The model under review builds one solid part; all positions refer to its coordinate system, in mm. Coordinates: 2 decimals unless noted, no trailing zeros. Loops run counter-clockwise (first coordinate to the right, second up) from the corner with the lowest first, then second, coordinate; pieces in that order, holes last. Notation, with made-up numbers: M -5,41 L 49,41 A31 cw 49,77 Z; hole C 21,20 d7. An arc over 180 degrees is marked long. Return JSON: item names as keys, results as strings.
```python
from build123d import *

# Parameters (mm, degrees)
SKETCH1_W           = 50
SKETCH1_H           = 23.75
BOSS_EXTRUDE1_DEPTH = 4
FILLET1_R           = 1.5
SKETCH2_R           = 1.8
CUT_EXTRUDE1_DEPTH  = 28.964542281


with BuildPart() as part:
    # Sketch1 → Boss-Extrude1 (new body)
    with BuildSketch(Plane.XY):
        Rectangle(SKETCH1_W, SKETCH1_H)
    extrude(amount=BOSS_EXTRUDE1_DEPTH)

    # Fillet1
    fillet1_edges = [part.edges().sort_by_distance(p)[0] for p in [
        (-25, 11.875, 2),
        (25, 11.875, 2),
    ]]
    fillet(fillet1_edges, radius=FILLET1_R)

    # Sketch2 → Cut-Extrude1 (cut, through all)
    with BuildSketch(Plane.XY.offset(4)):
        with Locations((-12.75, -1.625)):
            Circle(SKETCH2_R)
        with Locations((-20, 8.375)):
            Circle(SKETCH2_R)
        with Locations((12.75, -1.625)):
            Circle(SKETCH2_R)
        with Locations((20, 8.375)):
            Circle(SKETCH2_R)
    extrude(amount=-CUT_EXTRUDE1_DEPTH, mode=Mode.SUBTRACT)


solid = part.part
```
1. Add section B-B on z = 3.35. Give the boundary of the cut face in (x, y) (3 decimals), plus the area to 3 significant figures.
Check values:
{"outline": "M -25,-11.875 L 25,-11.875 L 25,10.375 A1.5 ccw 23.5,11.875 L -23.5,11.875 A1.5 ccw -25,10.375 Z; hole C -20,8.375 d3.6; hole C -12.75,-1.625 d3.6; hole C 12.75,-1.625 d3.6; hole C 20,8.375 d3.6", "area": "1,150 mm²"}
2. Add section D-D on x = -19. Give the boundary of the cut face in (y, z) (3 decimals).
Check values:
{"outline": "M -11.875,0 L 6.878,0 L 6.878,4 L -11.875,4 Z; M 9.872,0 L 11.875,0 L 11.875,4 L 9.872,4 Z"}
3. The part is to be moulded in two halves that separate along Y. For faces 1 (the face through (10.95, -1.55, 2.03)), 2 (the face through (0, 0, 4)), 3 (the face through (-24.572, 11.424, 2.028)), say which applies: released by +Y, released by -Y, zero draft, split by the parting line, or undercut.
Check values:
{"face 1": "undercut", "face 2": "zero draft", "face 3": "released by +Y"}
4. Add section A-A on x = 20. Give the boundary of the cut face in (y, z) (3 decimals).
Check values:
{"outline": "M -11.875,0 L 6.575,0 L 6.575,4 L -11.875,4 Z; M 10.175,0 L 11.875,0 L 11.875,4 L 10.175,4 Z"}
5. To check wall thickness, follow line 1 (X direction, y = 8.5, z = 2.9); line 2 (Y direction, x = 20, z = 2.1) (3 decimals); line 3 (X direction, y = -1.5, z = 2.05). State the ranges of each line that lie inside material, in increasing order.
Check values:
{"line 1": "-25 to -21.8, -18.2 to 18.2, 21.8 to 25", "line 2": "-11.875 to 6.575, 10.175 to 11.875", "line 3": "-25 to -14.55, -10.95 to 10.95, 14.55 to 25"}
6. Add section C-C on y = 9. Give the boundary of the cut face in (x, z).
Check values:
{"outline": "M -25,0 L -21.69,0 L -21.69,4 L -25,4 Z; M -18.31,0 L 18.31,0 L 18.31,4 L -18.31,4 Z; M 21.69,0 L 25,0 L 25,4 L 21.69,4 Z"}
